from build123d import *

# Parameters (mm, degrees)
SKETCH1_R             = 1
BOSS_EXTRUDE1_DEPTH   = 7
BOSS_EXTRUDE1_2_DEPTH = 7
SKETCH2_W             = 20.5
SKETCH2_H             = 10
BOSS_EXTRUDE2_DEPTH   = 2
SKETCH4_W             = 2
SKETCH4_H             = 10
BOSS_EXTRUDE3_DEPTH   = 6.5
FILLET1_SIZE          = 6
FILLET1_SIZE_2        = 0.3


with BuildPart() as part:
    # Sketch1 → Boss-Extrude1 (new body)
    with BuildSketch(Plane(origin=(0, 0, 0), x_dir=(0, 0, -1), z_dir=(1, 0, 0))):
        with Locations((-5, 0)):
            Circle(SKETCH1_R)
    extrude(amount=BOSS_EXTRUDE1_DEPTH)



with BuildPart() as body_2:
    # Sketch1 → Boss-Extrude1 2 (new body)
    with BuildSketch(Plane(origin=(0, 0, 0), x_dir=(0, 0, -1), z_dir=(1, 0, 0))):
        with Locations((5, 0)):
            Circle(SKETCH1_R)
    extrude(amount=BOSS_EXTRUDE1_2_DEPTH)


with BuildPart() as part_1:
    add(part.part)

    add(body_2.part)  # Boss-Extrude2 merges body 2
    # Sketch2 → Boss-Extrude2 (add)
    with BuildSketch(Plane.ZY):
        with Locations((0, -2.5)):
            Rectangle(SKETCH2_W, SKETCH2_H)
    extrude(amount=BOSS_EXTRUDE2_DEPTH)

    # Sketch4 → Boss-Extrude3 (add)
    with BuildSketch(Plane.ZY.offset(2)):
        with Locations((-11.25, -2.5)):
            Rectangle(SKETCH4_W, SKETCH4_H)
        with Locations((11.25, -2.5)):
            Rectangle(SKETCH4_W, SKETCH4_H)
    extrude(amount=-BOSS_EXTRUDE3_DEPTH)

    # Fillet1
    # an asymmetric fillet: 6, 0.3 mm, written as the material it takes off along each edge
    with BuildSketch(Plane(origin=(7, 0, -5), x_dir=(0, 0, -1), z_dir=(0, -1, 0))) as fillet1_piece_1:
        with BuildLine():
            Bezier((1, -FILLET1_SIZE), (1, 0), (1 - FILLET1_SIZE_2, 0), weights=[1, 0.707106781, 1])
            Line((1 - FILLET1_SIZE_2, 0), (1, 0))
            Line((1, 0), (1, -FILLET1_SIZE))
        make_face()
    revolve(axis=Axis((7, 0, -5), (1, 0, 0)), mode=Mode.SUBTRACT)
    with BuildSketch(Plane(origin=(7, 0, 5), x_dir=(0, 0, -1), z_dir=(0, -1, 0))) as fillet1_piece_2:
        with BuildLine():
            Bezier((1, -FILLET1_SIZE), (1, 0), (1 - FILLET1_SIZE_2, 0), weights=[1, 0.707106781, 1])
            Line((1 - FILLET1_SIZE_2, 0), (1, 0))
            Line((1, 0), (1, -FILLET1_SIZE))
        make_face()
    revolve(axis=Axis((7, 0, 5), (1, 0, 0)), mode=Mode.SUBTRACT)


solid = part_1.part
Geometry: final body of the model. Coordinates: model frame, mm. A direction names the side the tool comes from. Give positions to 0.01 mm unless a question says otherwise; leave off trailing zeros. Order: outer loops, then holes, each group sorted by start corner. A loop starts at its lowest first (then second) coordinate and runs counter-clockwise, first axis right, second up. Notation, with made-up numbers: (45, 49) - (75, 49) arc R18 ccw to (75, 83) - close; hole circle Ø7 at (-23.75, 30.5). An arc over 180 degrees is marked (long way). Use CSV: the item, a comma, the result in double quotes.
1. Section query B-B (z = -2). Output: boundary loops of the cut face in (x, y).
Answers below:
outline,"(-2, -7.5) - (0, -7.5) - (0, 2.5) - (-2, 2.5) - close"
2. Material intervals for line 1 along Z through (x, y) = (2.25, -4.5); line 2 along Z through (x, y) = (4, -0.5); line 3 along X through (y, z) = (1, -6.5), sorted ascending. Write a range as from..to.
Answers below:
line 1,"-12.25..-10.25, 10.25..12.25"
line 2,"-12.25..-10.25, -5.82..-4.18, 4.18..5.82, 10.25..12.25"
line 3,"-2..0"
3. Section query A-A (y = 1.5). Output: boundary loops of the cut face in (x, z).
Answers below:
outline,"(-2, -12.25) - (4.5, -12.25) - (4.5, -10.25) - (0, -10.25) - (0, 10.25) - (4.5, 10.25) - (4.5, 12.25) - (-2, 12.25) - close"
4. Contact query for flat-ended pins moving along their axis: pin 1 (3 mm diameter, centred on y = -2.5, z = 0, fed in from +X); pin 2 (5 mm diameter, centred on x = 4.5, z = 8.5, fed in from -Y); pin 3 (2 mm diameter, centred on y = -1.5, z = 11, fed in from +X); pin 4 (1 mm diameter, centred on x = 4, z = 4, fed in from +Y). Output: stop coordinate, or through.
Answers below:
pin 1,"x = 0"
pin 2,"y = -7.5"
pin 3,"x = 4.5"
pin 4,"y = 0.82"
5. Access query for faces 5 (the face through (2, -3, -10.25)), 6 (the face through (4.5, -2, 11)), 7 (the face through (4.5, -2, -11)). Directions: +Z, -Z, +X, -X, +Y, -Y. A direction counts if a zero-diameter tool reaches every point of the face in a straight line with its end or side. Return the directions, or none.
Answers below:
face 5,"+X, +Y, -Y"
face 6,"+Z, +X, +Y, -Y"
face 7,"-Z, +X, +Y, -Y"
6. Mould query, pull axis Z, two halves, no side actions, for faces 1 (the face through (0.5, -0.6, 5.8)), 2 (the face through (1, -3, 12.25)), 3 (the face through (-0.2, 2.5, -0.2)), 4 (the face through (2, -3, 10.25)). Classes: +Z half, -Z half, draft (parallel to the pull), parting line (faces both ways), or undercut.
Answers below:
face 1,"undercut"
face 2,"+Z half"
face 3,"draft"
face 4,"undercut"
